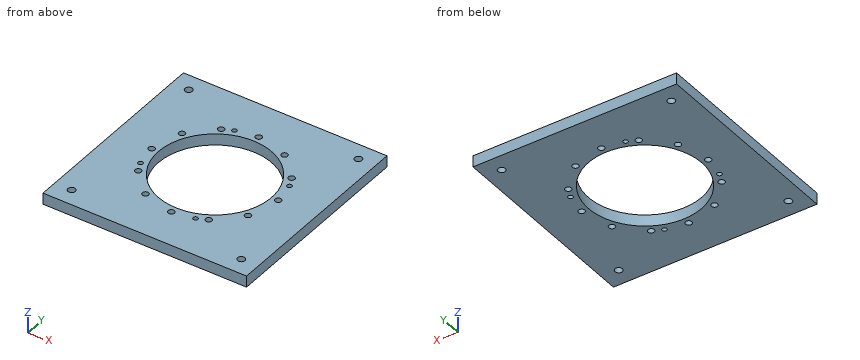
```python
from build123d import *

# Parameters (mm, degrees)
SKETCH_1_W          = 180
SKETCH_1_H          = 180
EXTRUDE_1_DEPTH     = 10
SKETCH_2_R          = 50
SKETCH_2_R_2        = 2.75
SKETCH_2_R_3        = 2.1
SKETCH_2_R_4        = 3.25
CUT_EXTRUDE_1_DEPTH = 11


with BuildPart() as part:
    # 草图1 → 凸台-拉伸1 (new body)
    with BuildSketch(Plane.XY):
        Rectangle(SKETCH_1_W, SKETCH_1_H)
    extrude(amount=EXTRUDE_1_DEPTH)

    # 草图2 → 切除-拉伸1 (cut)
    with BuildSketch(Plane(origin=(0, 0, 0), x_dir=(-1, 0, 0), z_dir=(0, 0, -1))):
        Circle(SKETCH_2_R)
        with Locations((-56, 0)):
            Circle(SKETCH_2_R_2)
        with Locations((-48.497422612, 28)):
            Circle(SKETCH_2_R_2)
        with Locations((-28, 48.497422612)):
            Circle(SKETCH_2_R_2)
        with Locations((0, 56)):
            Circle(SKETCH_2_R_2)
        with Locations((28, 48.497422612)):
            Circle(SKETCH_2_R_2)
        with Locations((48.497422612, 28)):
            Circle(SKETCH_2_R_2)
        with Locations((56, 0)):
            Circle(SKETCH_2_R_2)
        with Locations((48.497422612, -28)):
            Circle(SKETCH_2_R_2)
        with Locations((28, -48.497422612)):
            Circle(SKETCH_2_R_2)
        with Locations((0, -56)):
            Circle(SKETCH_2_R_2)
        with Locations((-28, -48.497422612)):
            Circle(SKETCH_2_R_2)
        with Locations((-48.497422612, -28)):
            Circle(SKETCH_2_R_2)
        with Locations((-52.622786764, 19.153128026)):
            Circle(SKETCH_2_R_3)
        with Locations((19.153128026, 52.622786764)):
            Circle(SKETCH_2_R_3)
        with Locations((52.622786764, -19.153128026)):
            Circle(SKETCH_2_R_3)
        with Locations((-19.153128026, -52.622786764)):
            Circle(SKETCH_2_R_3)
        with Locations((75, -75)):
            Circle(SKETCH_2_R_4)
        with Locations((75, 75)):
            Circle(SKETCH_2_R_4)
        with Locations((-75, -75)):
            Circle(SKETCH_2_R_4)
        with Locations((-75, 75)):
            Circle(SKETCH_2_R_4)
    extrude(amount=-CUT_EXTRUDE_1_DEPTH, mode=Mode.SUBTRACT)


solid = part.part
```
Input: part model. Units: mm. Frame: model coordinates. Give positions to 0.01 mm unless a question says otherwise; leave off trailing zeros. Write each loop counter-clockwise with the first axis right and the second up, starting at its lowest first coordinate (ties: lowest second). Pieces come first, ordered by that corner, then holes. Notation, with made-up numbers: (-11, 84.25) - (18, 84.25) arc R24 ccw to (18, 120.25) - close; hole circle Ø9 at (-28.5, 36). An arc over 180 degrees is marked (long way). Write item = value, one per line. Start each with the question number.
1) Cut plane A-A (y = -75). Return loops of the section in (x, z).
2) Pin query (flat end, axial travel): pin 1 (9 mm diameter, centred on x = 48.5, y = -28, fed in from -Z); pin 2 (3.5 mm diameter, centred on x = 28, y = 48.5, fed in from -Z). Return the tip coordinate at first contact, or that it passes through.
3) Cut plane B-B (x = 0). Return loops of the section in (y, z).
4) Material intervals for L1, parallel to Y at x = 75, z = 3.25; L2, parallel to Y at x = 0, z = 7.25; L3, parallel to Y at x = -56, z = 4.75, sorted ascending. Write a range as [from, to].
Answers follow:
q1.outline = (-90, 0) - (-78.25, 0) - (-78.25, 10) - (-90, 10) - close; (-71.75, 0) - (71.75, 0) - (71.75, 10) - (-71.75, 10) - close; (78.25, 0) - (90, 0) - (90, 10) - (78.25, 10) - close
q2.pin_1 = 0
q2.pin_2 = through
q3.outline = (-90, 0) - (-58.75, 0) - (-58.75, 10) - (-90, 10) - close; (-53.25, 0) - (-50, 0) - (-50, 10) - (-53.25, 10) - close; (50, 0) - (53.25, 0) - (53.25, 10) - (50, 10) - close; (58.75, 0) - (90, 0) - (90, 10) - (58.75, 10) - close
q4.L1 = [-90, -78.25], [-71.75, 71.75], [78.25, 90]
q4.L2 = [-90, -58.75], [-53.25, -50], [50, 53.25], [58.75, 90]
q4.L3 = [-90, -2.75], [2.75, 90]
